Check sheet for the drawn part. Datum: minimum x, y, z corner. Units: mm. A direction names the side the tool comes from. Round coordinates to 2 decimals unless told otherwise and drop trailing zeros. Order: outer loops, then holes, each group sorted by start corner. A loop starts at its lowest first (then second) coordinate and runs counter-clockwise, first axis right, second up. Notation, with made-up numbers: (-17.75, 13.25) - (16.25, 13.25) arc R12 ccw to (16.25, 30.25) - close; hole circle Ø10 at (63.5, -26). An arc over 180 degrees is marked (long way). Write each question's results on one line, items separated by ' | '.
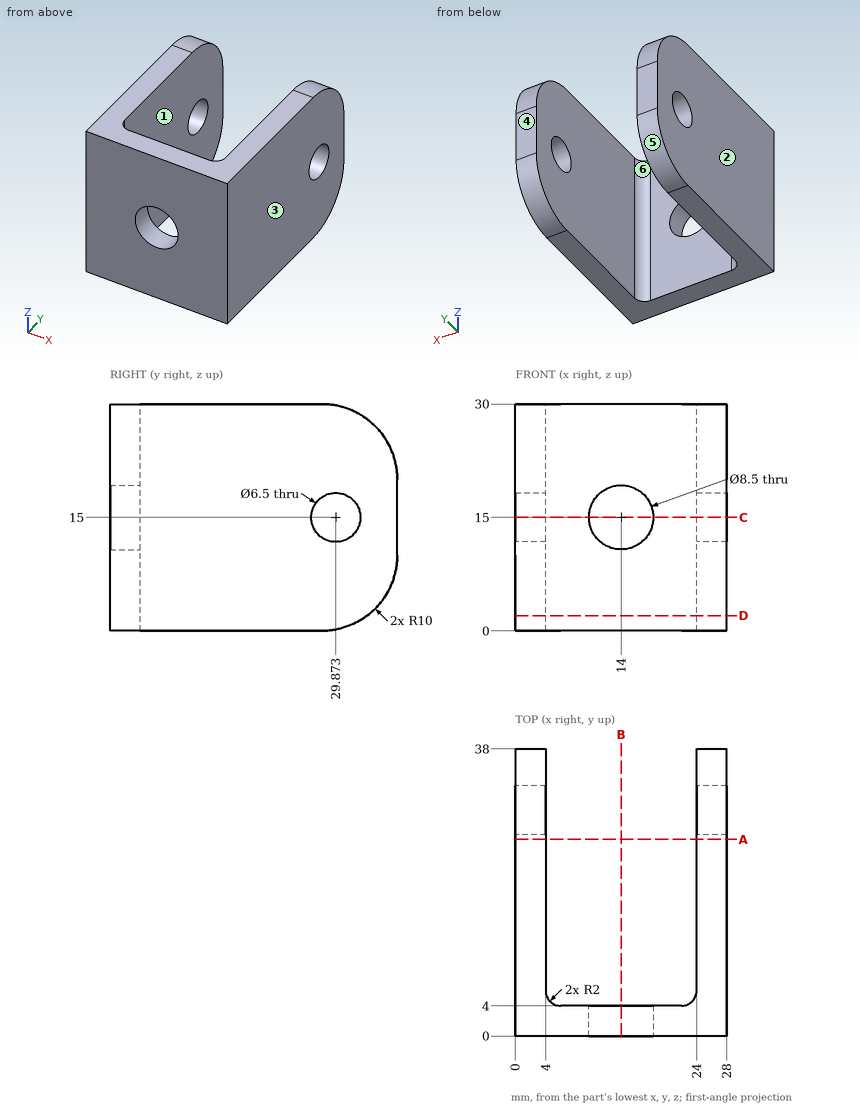
(1) Depth check by flat-ended pin: pin 1 Ø5 at (y, z) = (31.5, 15.5) entering from -X; pin 2 Ø13.5 at (x, z) = (14, 15) entering from +Y; pin 3 Ø13 at (x, z) = (17, 10) entering from +Y. Enter the tip coordinate at first touch or a pass-through.
Answers follow:
pin 1: x = 0 | pin 2: y = 4 | pin 3: y = 4.68
(2) Section check B-B (x = 14). Record the cut outline in (y, z), then the cut area to 3 significant figures.
Answers follow:
outline: (0, 0) - (4, 0) - (4, 10.75) - (0, 10.75) - close; (0, 19.25) - (4, 19.25) - (4, 30) - (0, 30) - close | area: 86.0 mm²
(3) Section check D-D (z = 2). Record the cut outline in (x, y).
Answers follow:
outline: (0, 0) - (28, 0) - (28, 34) - (24, 34) - (24, 6) arc R2 cw to (22, 4) - (6, 4) arc R2 cw to (4, 6) - (4, 34) - (0, 34) - close
(4) Section check C-C (z = 15). Record the cut outline in (x, y), then the cut area to 3 significant figures.
Answers follow:
outline: (0, 0) - (9.75, 0) - (9.75, 4) - (6, 4) arc R2 cw to (4, 6) - (4, 26.62) - (0, 26.62) - close; (0, 33.12) - (4, 33.12) - (4, 38) - (0, 38) - close; (18.25, 0) - (28, 0) - (28, 26.62) - (24, 26.62) - (24, 6) arc R2 cw to (22, 4) - (18.25, 4) - close; (24, 33.12) - (28, 33.12) - (28, 38) - (24, 38) - close | area: 300 mm²
(5) Material ranges on line 1 (X direction, y = 20, z = 9.75); line 2 (Z direction, x = 14, y = 1.6); line 3 (X direction, y = 2.8, z = 15), recorded low to high.
Answers follow:
line 1: 0 to 4, 24 to 28 | line 2: 0 to 10.75, 19.25 to 30 | line 3: 0 to 9.75, 18.25 to 28
(6) Access from +Z, -Z, +X, -X, +Y, -Y to the whole of each face (thin tool, end or side, straight path). Record for the marked faces 5 and 6.
Answers follow:
face 5: -Z, +X, -X, +Y | face 6: +Z, -Z, +Y
(7) Section check A-A (y = 26). Record the cut outline in (x, z), then the cut area to 3 significant figures.
Answers follow:
outline: (0, 0) - (4, 0) - (4, 30) - (0, 30) - close; (24, 0) - (28, 0) - (28, 30) - (24, 30) - close | area: 240 mm²
(8) Draft check along X on the marked faces 1, 2, 3 and 4. Enter one of: released by +X, released by -X, zero draft, split by the parting line, or undercut.
Answers follow:
face 1: undercut | face 2: released by -X | face 3: released by +X | face 4: zero draft
